Can you work these out from the model? Positions are in its coordinate system, mm. Face numbers are marked on the shaded views. Give positions to 0.01 mm unless a question says otherwise; leave off trailing zeros. Order: outer loops, then holes, each group sorted by start corner. A loop starts at its lowest first (then second) coordinate and runs counter-clockwise, first axis right, second up. Notation, with made-up numbers: M 20.25,61.25 L 45.25,61.25 A23 ccw 45.25,95.25 Z; hole C 28,-9.5 d9. An arc over 180 degrees is marked long. Answer as a JSON object with one key per item and string values.
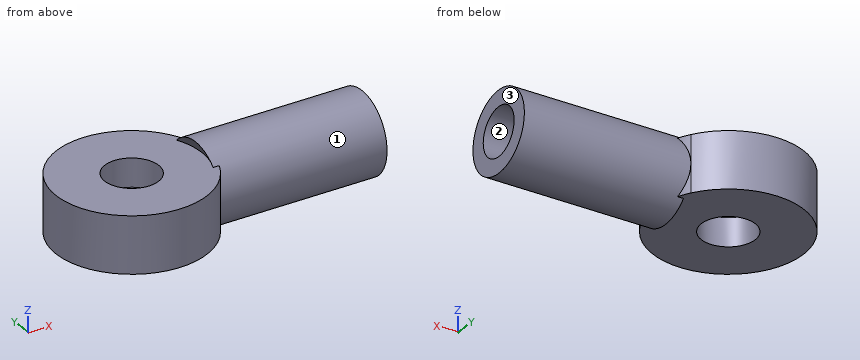
```python
from build123d import *

# Parameters (mm, degrees)
F0_R     = 5
F1_DEPTH = 5.25
F4_D     = 9
F4_DEPTH = 23
F4_TIP   = 2.7038727856


with BuildPart() as f1:
    # F0 (on Top) → F1 (new body, symmetric)
    with BuildSketch(Plane.XY):
        with BuildLine():
            ThreePointArc((11.8215904175, -7.5), (13.4443717935, -3.9049797794), (14, 0))
            ThreePointArc((14, 0), (13.4443717935, 3.9049797794), (11.8215904175, 7.5))
            ThreePointArc((11.8215904175, 7.5), (-14, 0), (11.8215904175, -7.5))
        make_face()
        Circle(F0_R, mode=Mode.SUBTRACT)
    extrude(amount=F1_DEPTH, both=True)

    # F0 (on Top) → F2 (revolve)
    with BuildSketch(Plane.XY):
        with BuildLine():
            ThreePointArc((11.8215904175, 7.5), (13.4443717935, 3.9049797794), (14, 0))
            Line((14, 0), (43, 0))
            Line((43, 0), (43, 7.5))
            Line((43, 7.5), (11.8215904175, 7.5))
        make_face()
    revolve(axis=Axis((18.6075619422, 0, 0), (-1, 0, 0)))

    # F4
    with Locations(Plane.YZ.offset(43)):
        with Locations((0, 0)):
            Hole(F4_D / 2, depth=F4_DEPTH)
            with Locations((0, 0, -(F4_DEPTH + F4_TIP / 2))):  # 118° drill point
                Cone(0, F4_D / 2, F4_TIP, mode=Mode.SUBTRACT)


solid = f1.part
```
1) I want a section at B-B on y = -6.75. Write out the boundary of the cut face in (x, z), and give its area (3 significant figures).
Results found:
{"outline": "M -12.27,-5.25 L 12.27,-5.25 L 12.27,-3.27 L 43,-3.27 L 43,3.27 L 12.27,3.27 L 12.27,5.25 L -12.27,5.25 Z", "area": "459 mm²"}
2) I want a section at C-C on x = 29.5. Write out the boundary of the cut face in (y, z).
Results found:
{"outline": "C 0,0 d15; hole C 0,0 d9"}
3) I need wall thicknesses on L1, parallel to Z at x = 28, y = 0; L2, parallel to Y at x = 0, z = -3.1; L3, parallel to Z at x = 19.5, y = 1.75. Which ranges of each line are inside material? Lowest first, please.
Results found:
{"L1": "z = -7.5 to -4.5, 4.5 to 7.5", "L2": "y = -14 to -5, 5 to 14", "L3": "z = -7.29 to -3.22, 3.22 to 7.29"}
4) I'm going to push flat-ended pins straight in: pin 1 Ø8 at (y, z) = (-7.5, -3.5) entering from -X; pin 2 Ø5 at (y, z) = (-5.5, 0.5) entering from -X; pin 3 Ø4 at (x, z) = (3.5, 6) entering from +Y. Where does each tip first touch, or does it pass through?
Results found:
{"pin 1": "stops at x = -13.56", "pin 2": "stops at x = -13.67", "pin 3": "stops at y = 13.9"}
5) I want a section at A-A on x = 0. Write out the boundary of the cut face in (y, z).
Results found:
{"outline": "M -14,-5.25 L -5,-5.25 L -5,5.25 L -14,5.25 Z; M 5,-5.25 L 14,-5.25 L 14,5.25 L 5,5.25 Z"}
6) I want a section at D-D on x = -9. Write out the boundary of the cut face in (y, z), and give its area (3 significant figures).
Results found:
{"outline": "M -10.72,-5.25 L 10.72,-5.25 L 10.72,5.25 L -10.72,5.25 Z", "area": "225 mm²"}
7) Thinking about a two-plate mould opening in Z: for the marked faces 1, 2 and 3, which applies, pulls with the +Z half, pulls with the -Z half, needs draft (parallel to the pull), parting line crosses it, or undercut?
Results found:
{"face 1": "parting line crosses it", "face 2": "undercut", "face 3": "needs draft"}
